from build123d import *

# Parameters (mm, degrees)
SKETCH1_R           = 0.6096
SKETCH1_R_2         = 0.5715
BOSS_EXTRUDE1_DEPTH = 1.5875


with BuildPart() as part:
    # Sketch1 → Boss-Extrude1 (new body)
    with BuildSketch(Plane.XY):
        with BuildLine():
            Line((30.48, -22.225), (29.415104476, -11.9888))
            ThreePointArc((29.415104476, -11.9888), (28.715873825, 1.490040556), (26.625688573, 14.824176893))
            ThreePointArc((26.625688573, 14.824176893), (23.941924767, 20.101731209), (18.415, 22.225))
            Line((18.415, 22.225), (-18.415, 22.225))
            ThreePointArc((-18.415, 22.225), (-23.941924767, 20.101731209), (-26.625688573, 14.824176893))
            ThreePointArc((-26.625688573, 14.824176893), (-28.715873825, 1.490040556), (-29.415104476, -11.9888))
            Line((-29.415104476, -11.9888), (-30.48, -22.225))
            Line((-30.48, -22.225), (30.48, -22.225))
        make_face()
        with BuildLine():
            ThreePointArc((17.725268352, 19.939), (19.155271645, 17.728799653), (21.365471992, 19.158802947))
            ThreePointArc((21.365471992, 19.158802947), (23.441797038, 17.188737724), (24.362294321, 14.478577686))
            ThreePointArc((24.362294321, 14.478577686), (26.441646573, 1.258286409), (27.129050016, -12.106865432))
            Line((27.129050016, -12.106865432), (27.943845061, -19.939))
            Line((27.943845061, -19.939), (21.489528855, -19.939))
            ThreePointArc((21.489528855, -19.939), (19.457528855, -17.907), (17.425528855, -19.939))
            Line((17.425528855, -19.939), (-17.425528855, -19.939))
            ThreePointArc((-17.425528855, -19.939), (-19.457528855, -17.907), (-21.489528855, -19.939))
            Line((-21.489528855, -19.939), (-27.943845061, -19.939))
            Line((-27.943845061, -19.939), (-27.129050016, -12.106865432))
            ThreePointArc((-27.129050016, -12.106865432), (-26.441646573, 1.258286409), (-24.362294321, 14.478577686))
            ThreePointArc((-24.362294321, 14.478577686), (-23.441797038, 17.188737724), (-21.365471992, 19.158802947))
            ThreePointArc((-21.365471992, 19.158802947), (-19.155271645, 17.728799653), (-17.725268352, 19.939))
            Line((-17.725268352, 19.939), (17.725268352, 19.939))
        make_face(mode=Mode.SUBTRACT)
        with Locations((19.457528855, 19.05)):
            Circle(SKETCH1_R, mode=Mode.SUBTRACT)
        with Locations((-19.457528855, 19.05)):
            Circle(SKETCH1_R, mode=Mode.SUBTRACT)
        with Locations((19.457528855, -19.05)):
            Circle(SKETCH1_R_2, mode=Mode.SUBTRACT)
        with Locations((-19.457528855, -19.05)):
            Circle(SKETCH1_R_2, mode=Mode.SUBTRACT)
    extrude(amount=BOSS_EXTRUDE1_DEPTH)


solid = part.part
Verification items for the finished model (mm, model axes). A direction names the side the tool comes from. Coordinates: 2 decimals unless noted, no trailing zeros. Loops run counter-clockwise (first coordinate to the right, second up) from the corner with the lowest first, then second, coordinate; pieces in that order, holes last. Notation, with made-up numbers: (60.5, -2.5) -> (70.5, -2.5) arc R12 ccw to (70.5, 9.5) -> close; hole circle Ø2 at (63, 81.25). An arc over 180 degrees is marked (long way). Answer as a JSON object with one key per item and string values. Group by question number.
Item 1: Sectioned sample at B-B on z = 1.05. State how many separate pieces and enclosed holes the cut face has, plus the area to 3 significant figures.
Item 2: Sectioned sample at C-C on y = -16.5. Record the boundary of the cut face in (x, z).
Item 3: Sectioned sample at A-A on x = -4. Record the boundary of the cut face in (y, z) (1 decimal).
Item 4: Mould release check, pull along Y, two halves, no side actions. Record for faces 1 (the flat face through (-29.94, -17.04, 0.78)), 2 (the cylindrical face through (-23.464, 17.155, 0.783)), 3 (the flat face through (0, -22.225, 1)): +Y half, -Y half, draft (parallel to the pull), parting line (faces both ways), or undercut.
Item 5: Tool access check on faces 4 (the cylindrical face through (24.005, 20.045, 0.783)), 5 (the cylindrical face through (-19.413, -17.907, 0.783)). Record the directions out of +Z, -Z, +X, -X, +Y, -Y that give a thin tool (end or side, any length) a straight path to the whole face; none if there is none.
Item 6: Scan lines: probe 1 along Y at (x, z) = (10, 1.05) (3 decimals); probe 2 along Y at (x, z) = (21, 0.55) (3 decimals); probe 3 along X at (y, z) = (11, 0.85). Record each from-to range of solid material in increasing order.
Evaluation:
{
 "1": {"separate pieces": "1", "enclosed holes": "5", "area": "451 mm²"},
 "2": {"outline": "(-29.88, 0) -> (-27.59, 0) -> (-27.59, 1.59) -> (-29.88, 1.59) -> close; (27.59, 0) -> (29.88, 0) -> (29.88, 1.59) -> (27.59, 1.59) -> close"},
 "3": {"outline": "(-22.2, 0) -> (-19.9, 0) -> (-19.9, 1.6) -> (-22.2, 1.6) -> close; (19.9, 0) -> (22.2, 0) -> (22.2, 1.6) -> (19.9, 1.6) -> close"},
 "4": {"face 1": "+Y half", "face 2": "undercut", "face 3": "-Y half"},
 "5": {"face 4": "+Z, -Z, +X, +Y", "face 5": "+Z, -Z"},
 "6": {"probe 1": "y = -22.225 to -19.939, 19.939 to 22.225", "probe 2": "y = -22.225 to -18.616, 18.387 to 21.81", "probe 3": "x = -27.37 to -25.05, 25.05 to 27.37"}
}
